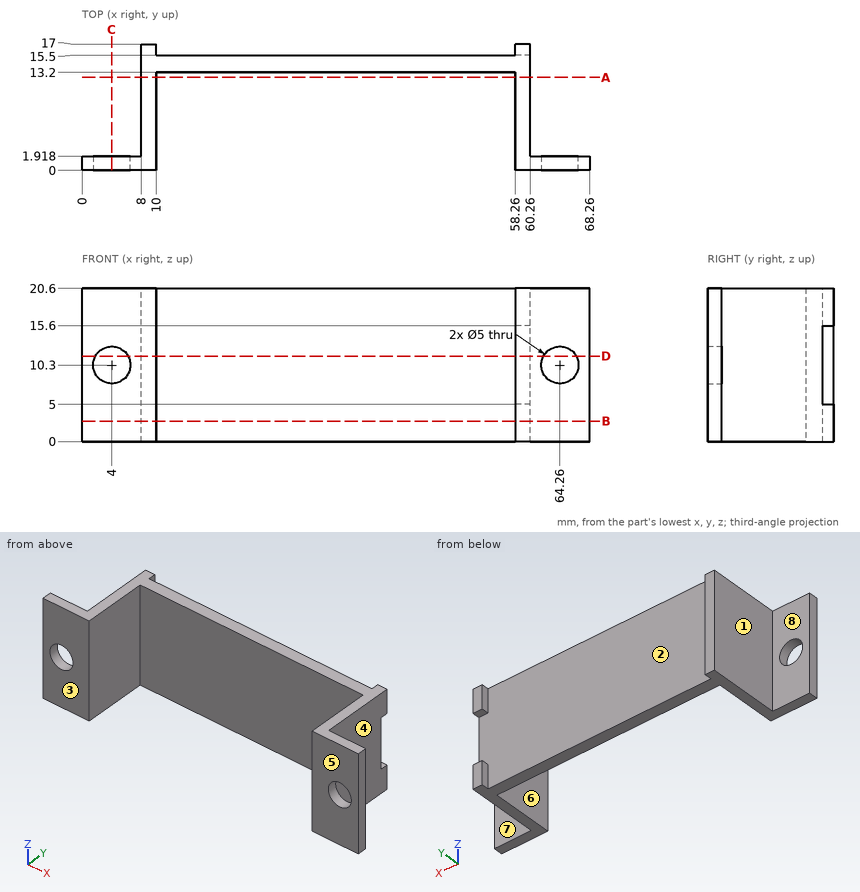
Geometry: see drawing. Coordinates: mm, zero at the bounding-box minimum. A direction names the side the tool comes from. Give positions to 0.01 mm unless a question says otherwise; leave off trailing zeros. Loops run counter-clockwise (first coordinate to the right, second up) from the corner with the lowest first, then second, coordinate; pieces in that order, holes last. Notation, with made-up numbers: (39, 53) - (74, 53) arc R25 cw to (74, 67) - close; hole circle Ø5 at (3.25, 14). An arc over 180 degrees is marked (long way). Answer as CSV lines item,"result". Start each with the question number.
1. Section A-A, the plane y = 12.5. Return loops of the section in (x, z).
2. Draft query along X for the marked faces 1, 2, 3 and 4. Return one class per face: released by +X, released by -X, zero draft, split by the parting line, or undercut.
3. Ray query, L1, parallel to Z at x = 64.26, y = 1.25; L2, parallel to X at y = 6.25, z = 5.5; L3, parallel to Y at x = 55.5, z = 9.25. Return the intervals inside material, ascending.
4. Reachability of the marked faces 5, 6, 7 and 8 from +Z, -Z, +X, -X, +Y, -Y: full face, straight path, thin tool, end or side. Return the list, or none.
5. Section C-C, the plane x = 4. Return loops of the section in (y, z).
6. Section B-B, the plane z = 2.75. Return loops of the section in (x, y).
7. Section D-D, the plane z = 11.5. Return loops of the section in (x, y), plus the area to 3 significant figures.
8. Pin query (flat end, axial travel): P1, Ø7.5, axis at y = 6.5, z = 13.5, coming from the -X side; P2, Ø1.5, axis at y = 7.5, z = 6.5, coming from the +X side; P3, Ø6, axis at x = 24, z = 13.5, coming from the +Y side. Return the tip coordinate at first contact, or that it passes through.
Answers:
1,outline,"(8, 0) - (10, 0) - (10, 20.6) - (8, 20.6) - close; (58.26, 0) - (60.26, 0) - (60.26, 20.6) - (58.26, 20.6) - close"
2,face 1,"released by -X"
2,face 2,"undercut"
2,face 3,"zero draft"
2,face 4,"released by +X"
3,L1,"z = 0 to 7.8, 12.8 to 20.6"
3,L2,"x = 8 to 10, 58.26 to 60.26"
3,L3,"y = 13.2 to 15.5"
4,face 5,"+Z, -Z, +X, -X, -Y"
4,face 6,"+Z, -Z, -Y"
4,face 7,"+Z, -Z, +X, +Y"
4,face 8,"+Z, -Z, -X, +Y"
5,outline,"(0, 0) - (1.92, 0) - (1.92, 7.8) - (0, 7.8) - close; (0, 12.8) - (1.92, 12.8) - (1.92, 20.6) - (0, 20.6) - close"
6,outline,"(0, 0) - (10, 0) - (10, 13.2) - (58.26, 13.2) - (58.26, 0) - (68.26, 0) - (68.26, 1.92) - (60.26, 1.92) - (60.26, 17) - (58.26, 17) - (58.26, 15.5) - (10, 15.5) - (10, 17) - (8, 17) - (8, 1.92) - (0, 1.92) - close"
7,outline,"(0, 0) - (1.81, 0) - (1.81, 1.92) - (0, 1.92) - close; (6.19, 0) - (10, 0) - (10, 13.2) - (58.26, 13.2) - (58.26, 0) - (62.07, 0) - (62.07, 1.92) - (60.26, 1.92) - (60.26, 15.5) - (10, 15.5) - (10, 17) - (8, 17) - (8, 1.92) - (6.19, 1.92) - close; (66.45, 0) - (68.26, 0) - (68.26, 1.92) - (66.45, 1.92) - close"
7,area,"190 mm2"
8,P1,"stops at x = 8"
8,P2,"stops at x = 60.26"
8,P3,"stops at y = 15.5"
